Study the drawing (mm; zero at the part's minimum x, y, z) and answer. Coordinates: 2 decimals unless noted, no trailing zeros. Write each loop counter-clockwise with the first axis right and the second up, starting at its lowest first coordinate (ties: lowest second). Pieces come first, ordered by that corner, then holes. Notation, with made-up numbers: (84.25, -33) - (130.25, -33) arc R32 cw to (130.25, 2) - close; hole circle Ø4 at (86, 34). An arc over 180 degrees is marked (long way). One line per item, written item: value.
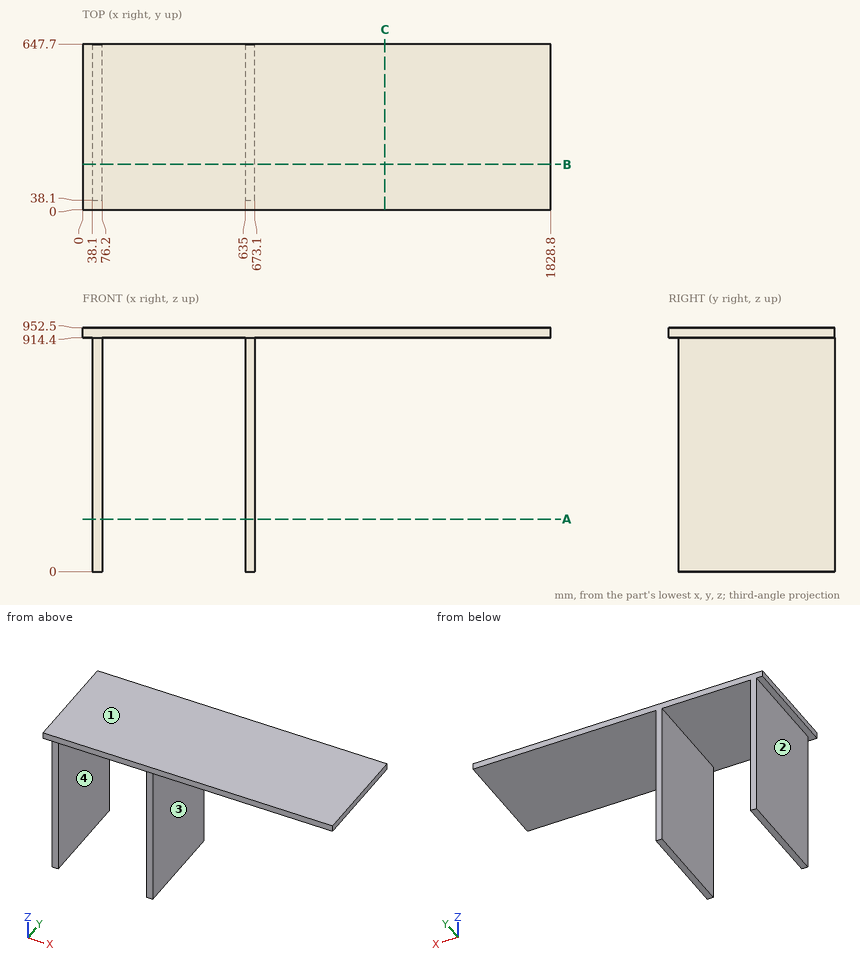
Item 1: Section C-C, the plane x = 1181.5 is taken. Determine the outline of the cut face in (y, z).
Evaluation:
outline: (0, 914.4) - (647.7, 914.4) - (647.7, 952.5) - (0, 952.5) - close
Item 2: Section A-A, the plane z = 205.5 is taken. Determine the outline of the cut face in (x, y).
Evaluation:
outline: (38.1, 38.1) - (76.2, 38.1) - (76.2, 647.7) - (38.1, 647.7) - close; (635, 38.1) - (673.1, 38.1) - (673.1, 647.7) - (635, 647.7) - close
Item 3: Section B-B, the plane y = 177.5 is taken. Determine the outline of the cut face in (x, z), then the cut area to 3 significant figures.
Evaluation:
outline: (0, 914.4) - (38.1, 914.4) - (38.1, 0) - (76.2, 0) - (76.2, 914.4) - (635, 914.4) - (635, 0) - (673.1, 0) - (673.1, 914.4) - (1828.8, 914.4) - (1828.8, 952.5) - (0, 952.5) - close
area: 139,000 mm2
Item 4: Determine the mould class of the marked faces 1, 2, 3 and 4 for opening direction X: +X half, -X half, draft (parallel to the pull), parting line (faces both ways), or undercut.
Evaluation:
face 1: draft
face 2: -X half
face 3: +X half
face 4: undercut
Item 5: Given pin 1 (6 mm diameter, centred on y = 185.5, z = 507, fed in from -X); pin 2 (8 mm diameter, centred on x = 832, y = 364.5, fed in from -Z), each flat-ended and moving along its own axis, determine where each tip first touches the part or whether it passes through.
Evaluation:
pin 1: stops at x = 38.1
pin 2: stops at z = 914.4
Item 6: Consider probe 1 along X at (y, z) = (484, 726.5); probe 2 along Z at (x, y) = (817.5, 217.5). Determine where each line is inside the solid, lowest interval first.
Evaluation:
probe 1: x = 38.1 to 76.2, 635 to 673.1
probe 2: z = 914.4 to 952.5
